The model under review builds one solid part; all positions refer to its coordinate system, in mm. A direction names the side the tool comes from. Coordinates: 2 decimals unless noted, no trailing zeros. Write each loop counter-clockwise with the first axis right and the second up, starting at its lowest first coordinate (ties: lowest second). Pieces come first, ordered by that corner, then holes.
```python
from build123d import *

# Parameters (mm, degrees)
F1_DEPTH      = 19.05
F2_W          = 254
F2_H          = 50.8
F3_DEPTH      = 133.35
F5_R          = 44.45
F6_DEPTH      = 19.051
F7_DEPTH      = 107.95
F8_DEPTH      = 133.351
F8_DEPTH_BACK = 19.051
F10_DEPTH     = 88.9


with BuildPart() as f1:
    # F0 (on Front) → F1 (new body)
    with BuildSketch(Plane.XZ):
        with BuildLine():
            Line((0, 50.8), (0, 0))
            Line((0, 0), (254, 0))
            Line((254, 0), (254, 50.8))
            Line((254, 50.8), (184.82177, 203.2))
            ThreePointArc((184.82177, 203.2), (127, 240.45323), (69.17823, 203.2))
            Line((69.17823, 203.2), (0, 50.8))
        make_face()
    extrude(amount=F1_DEPTH)

    # F2 (on face) → F3 (join)
    with BuildSketch(Plane.XZ.offset(19.05)):
        with Locations((127, 25.4)):
            Rectangle(F2_W, F2_H)
    extrude(amount=F3_DEPTH)

    # F5 (on face) → F6 (cut, through all)
    with BuildSketch(Plane.XZ.offset(19.05)):
        with Locations((127, 176.95323)):
            Circle(F5_R)
    extrude(amount=-F6_DEPTH, mode=Mode.SUBTRACT)

    # F4 (on face) → F7 (join)
    with BuildSketch(Plane.XZ.offset(19.05)):
        with BuildLine():
            ThreePointArc((69.17823, 203.2), (113.57302, 114.88902), (190.5, 176.95323))
            ThreePointArc((190.5, 176.95323), (189.06421, 190.380211), (184.82177, 203.2))
            ThreePointArc((184.82177, 203.2), (127, 240.45323), (69.17823, 203.2))
        make_face()
    extrude(amount=F7_DEPTH)

    # F5 (on face) → F8 (cut, two sides)
    with BuildSketch(Plane.XZ.offset(19.05)) as f8_sk:
        with Locations((127, 176.95323)):
            Circle(F5_R)
    extrude(amount=F8_DEPTH, mode=Mode.SUBTRACT)
    extrude(f8_sk.sketch, amount=-F8_DEPTH_BACK, mode=Mode.SUBTRACT)

    # F9 (on face) → F10 (join)
    with BuildSketch(Plane.XZ.offset(19.05)):
        with BuildLine():
            Line((117.475, 114.17167), (117.475, 50.8))
            Line((117.475, 50.8), (136.525, 50.8))
            Line((136.525, 50.8), (136.525, 114.17167))
            ThreePointArc((136.525, 114.17167), (127, 113.45323), (117.475, 114.17167))
        make_face()
    extrude(amount=F10_DEPTH)


solid = f1.part
```
Item 1: Mouldability with a two-part tool opening along Z and no side actions: class faces 1 (the face through (219.895, -9.392, 125.933)), 2 (the face through (125, -75, 0)), 3 (the face through (194, -19.05, 94)), 4 (the face through (125, -152.4, 26)) as pulls with the +Z half, pulls with the -Z half, needs draft (parallel to the pull), parting line crosses it, or undercut.
Solved:
face 1: pulls with the +Z half
face 2: pulls with the -Z half
face 3: undercut
face 4: needs draft
Item 2: Machinability: for faces 5 (the face through (71, -19.05, 94)), 6 (the face through (140, -127, 220)), 7 (the face through (125, -114, 50.8)), 8 (the face through (136.525, -63, 82)), which of the approach directions +Z, -Z, +X, -X, +Y, -Y give a long, thin tool a straight path to every point of the face, cutting with its end or side? Answer none if there is none.
Solved:
face 5: -X, -Y
face 6: +Z, +X, -X, -Y
face 7: -Y
face 8: +X, -Y
Item 3: Take a section at C-C, the plane y = -53. Write out the cut boundary in (x, z) (3 decimals), plus the area to 3 significant figures.
Solved:
outline: (0, 0) - (254, 0) - (254, 50.8) - (136.525, 50.8) - (136.525, 114.172) arc R63.5 ccw to (190.5, 176.953) arc R63.5 ccw to (184.822, 203.2) arc R63.5 ccw (long way) to (117.475, 114.172) - (117.475, 50.8) - (0, 50.8) - close; hole circle Ø88.9 at (127, 176.953)
area: 20,600 mm2
Item 4: Take a section at D-D, the plane z = 145.5. Write out the cut boundary in (x, y), plus the area to 3 significant figures.
Solved:
outline: (42.99, -19.05) - (71.84, -19.05) - (71.84, -127) - (95.59, -127) - (95.59, 0) - (42.99, 0) - close; (158.41, -127) - (182.16, -127) - (182.16, -19.05) - (211.01, -19.05) - (211.01, 0) - (158.41, 0) - close
area: 7,130 mm2
Item 5: Take a section at A-A, the plane x = 127. Write out the cut boundary in (y, z), plus the area to 3 significant figures.
Solved:
outline: (-152.4, 0) - (0, 0) - (0, 132.5) - (-127, 132.5) - (-127, 113.45) - (-107.95, 113.45) - (-107.95, 50.8) - (-152.4, 50.8) - close; (-127, 221.4) - (0, 221.4) - (0, 240.45) - (-127, 240.45) - close
area: 19,300 mm2
Item 6: To check wall thickness, follow line 1 along Z through (x, y) = (128, -124.5); line 2 along Z through (x, y) = (127, -49); line 3 along Z through (x, y) = (92.5, -49.5). State the ranges of each line that lie inside material, in increasing order.
Solved:
line 1: z = 0 to 50.8, 113.46 to 132.51, 221.39 to 240.45
line 2: z = 0 to 132.5, 221.4 to 240.45
line 3: z = 0 to 50.8, 123.64 to 148.93, 204.98 to 230.26
Item 7: Take a section at B-B, the plane y = -123. Write out the cut boundary in (x, z), plus the area to 3 significant figures.
Solved:
outline: (0, 0) - (254, 0) - (254, 50.8) - (0, 50.8) - close; (184.82, 203.2) arc R63.5 ccw (long way) to (190.5, 176.95) arc R63.5 ccw to start; hole circle Ø88.9 at (127, 176.95)
area: 19,400 mm2
Item 8: For pin 1 (19 mm diameter, centred on y = -49, z = 89, fed in from -X) (3 decimals); pin 2 (3 mm diameter, centred on x = 90.5, z = 93.5, fed in from -Y); pin 3 (1 mm diameter, centred on y = -117.5, z = 118, fed in from +X), all flat-tipped, find the tip position at first contact; note any pin that passes through.
Solved:
pin 1: stops at x = 117.475
pin 2: stops at y = -19.05
pin 3: stops at x = 151.81
